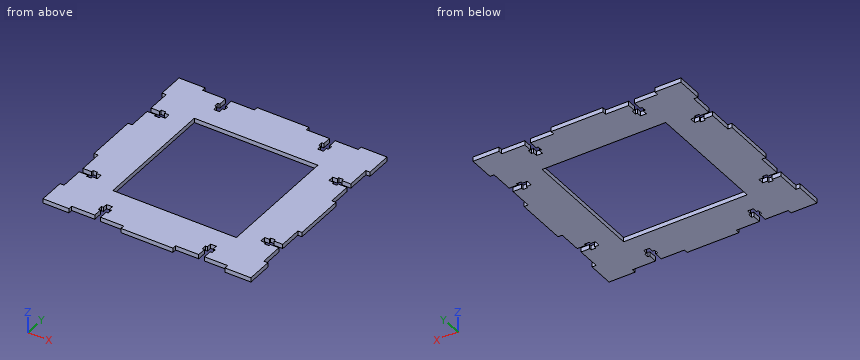
from build123d import *

# Parameters (mm, degrees)
SKETCH1_W           = 89.973098965
SKETCH1_H           = 90.646237782
BOSS_EXTRUDE1_DEPTH = 3.175


with BuildPart() as part:
    # Sketch1 → Boss-Extrude1 (new body)
    with BuildSketch(Plane.XY):
        Polygon((0, 154.39750188), (0, 135.470394989), (2.980646754, 135.470394989), (2.980646754, 118.65457955), (9.289682385, 118.65457955), (9.289682385, 120.144902927), (12.717426152, 120.144902927), (12.717426152, 118.65457955), (16.14516992, 118.65457955), (16.14516992, 114.431996648), (12.717426152, 114.431996648), (12.717426152, 112.94167327), (9.289682385, 112.94167327), (9.289682385, 114.431996648), (2.980646754, 114.431996648), (2.980646754, 97.616181208), (0, 97.616181208), (0, 59.761967427), (2.980646754, 59.761967427), (2.980646754, 42.946151987), (9.289682385, 42.946151987), (9.289682385, 44.436475364), (12.717426152, 44.436475364), (12.717426152, 42.946151987), (16.14516992, 42.946151987), (16.14516992, 38.723569085), (12.717426152, 38.723569085), (12.717426152, 37.233245708), (9.289682385, 37.233245708), (9.289682385, 38.723569085), (2.980646754, 38.723569085), (2.980646754, 21.907753645), (0, 21.907753645), (0, 2.980646754), (18.927106891, 2.980646754), (18.927106891, 5.961293509), (35.74292233, 5.961293509), (35.74292233, 12.270329139), (34.252598953, 12.270329139), (34.252598953, 15.698072907), (35.74292233, 15.698072907), (35.74292233, 19.125816674), (39.965505232, 19.125816674), (39.965505232, 15.698072907), (41.45582861, 15.698072907), (41.45582861, 12.270329139), (39.965505232, 12.270329139), (39.965505232, 5.961293509), (56.781320672, 5.961293509), (56.781320672, 2.980646754), (94.635534454, 2.980646754), (94.635534454, 5.961293509), (111.451349893, 5.961293509), (111.451349893, 12.270329139), (109.961026516, 12.270329139), (109.961026516, 15.698072907), (111.451349893, 15.698072907), (111.451349893, 19.125816674), (115.673932795, 19.125816674), (115.673932795, 15.698072907), (117.164256172, 15.698072907), (117.164256172, 12.270329139), (115.673932795, 12.270329139), (115.673932795, 5.961293509), (132.489748235, 5.961293509), (132.489748235, 2.980646754), (151.416855126, 2.980646754), (151.416855126, 21.907753645), (148.436208371, 21.907753645), (148.436208371, 38.723569085), (142.127172741, 38.723569085), (142.127172741, 37.233245708), (138.699428973, 37.233245708), (138.699428973, 38.723569085), (135.271685206, 38.723569085), (135.271685206, 42.946151987), (138.699428973, 42.946151987), (138.699428973, 44.436475364), (142.127172741, 44.436475364), (142.127172741, 42.946151987), (148.436208371, 42.946151987), (148.436208371, 59.761967427), (151.416855126, 59.761967427), (151.416855126, 97.616181208), (148.436208371, 97.616181208), (148.436208371, 114.431996648), (142.127172741, 114.431996648), (142.127172741, 112.94167327), (138.699428973, 112.94167327), (138.699428973, 114.431996648), (135.271685206, 114.431996648), (135.271685206, 118.65457955), (138.699428973, 118.65457955), (138.699428973, 120.144902927), (142.127172741, 120.144902927), (142.127172741, 118.65457955), (148.436208371, 118.65457955), (148.436208371, 135.470394989), (151.416855126, 135.470394989), (151.416855126, 154.39750188), (132.489748235, 154.39750188), (132.489748235, 151.416855126), (115.673932795, 151.416855126), (115.673932795, 145.107819495), (117.164256172, 145.107819495), (117.164256172, 141.680075728), (115.673932795, 141.680075728), (115.673932795, 138.25233196), (111.451349893, 138.25233196), (111.451349893, 141.680075728), (109.961026516, 141.680075728), (109.961026516, 145.107819495), (111.451349893, 145.107819495), (111.451349893, 151.416855126), (94.635534454, 151.416855126), (94.635534454, 154.39750188), (56.781320672, 154.39750188), (56.781320672, 151.416855126), (39.965505232, 151.416855126), (39.965505232, 145.107819495), (41.45582861, 145.107819495), (41.45582861, 141.680075728), (39.965505232, 141.680075728), (39.965505232, 138.25233196), (35.74292233, 138.25233196), (35.74292233, 141.680075728), (34.252598953, 141.680075728), (34.252598953, 145.107819495), (35.74292233, 145.107819495), (35.74292233, 151.416855126), (18.927106891, 151.416855126), (18.927106891, 154.39750188), align=None)
        with Locations((75.89557754, 78.791987571)):
            Rectangle(SKETCH1_W, SKETCH1_H, mode=Mode.SUBTRACT)
    extrude(amount=BOSS_EXTRUDE1_DEPTH)


solid = part.part
CAD build for the part. Positions are in the model's coordinates, mm. Round coordinates to 2 decimals unless told otherwise and drop trailing zeros. Loops run counter-clockwise (first coordinate to the right, second up) from the corner with the lowest first, then second, coordinate; pieces in that order, holes last. Notation, with made-up numbers: (-32, -39.5) - (22, -39.5) arc R13 cw to (22, -15.5) - close; hole circle Ø10 at (64.25, 65.25). An arc over 180 degrees is marked (long way). Put each result on its own line as item: value.
1. Pin check, flat tips, straight feed: P1, Ø1.6, axis at x = 126, z = 1, coming from the -Y side; P2, Ø0.7, axis at x = 116.5, z = 2, coming from the +Y side; P3, Ø1, axis at y = 40, z = 1, coming from the +X side. Stop position of each tip, or through.
Geometry check:
P1: y = 5.96
P2: y = 151.42
P3: x = 135.27
2. Wall check: line 1 (Y direction, x = 140.5, z = 2.3); line 2 (X direction, y = 142, z = 0.4); line 3 (X direction, y = 18.5, z = 0.9). Give the ranges that are in metal, low to high.
Geometry check:
line 1: 2.98 to 37.23, 44.44 to 112.94, 120.14 to 154.4
line 2: 0 to 34.25, 41.46 to 109.96, 117.16 to 151.42
line 3: 0 to 35.74, 39.97 to 111.45, 115.67 to 151.42
3. Slice it at C-C on x = 125.5. List the corners of the cut face in (y, z) (3 decimals).
Geometry check:
outline: (5.961, 0) - (151.417, 0) - (151.417, 3.175) - (5.961, 3.175) - close
4. Slice it at B-B on y = 65. List the corners of the cut face in (x, z) (3 decimals), and give its area (3 significant figures).
Geometry check:
outline: (0, 0) - (30.909, 0) - (30.909, 3.175) - (0, 3.175) - close; (120.882, 0) - (151.417, 0) - (151.417, 3.175) - (120.882, 3.175) - close
area: 195 mm²
5. Slice it at D-D on y = 132. List the corners of the cut face in (x, z) (3 decimals), and give its area (3 significant figures).
Geometry check:
outline: (2.981, 0) - (148.436, 0) - (148.436, 3.175) - (2.981, 3.175) - close
area: 462 mm²
6. Slice it at A-A on x = 51. List the corners of the cut face in (y, z) (3 decimals).
Geometry check:
outline: (5.961, 0) - (33.469, 0) - (33.469, 3.175) - (5.961, 3.175) - close; (124.115, 0) - (151.417, 0) - (151.417, 3.175) - (124.115, 3.175) - close
